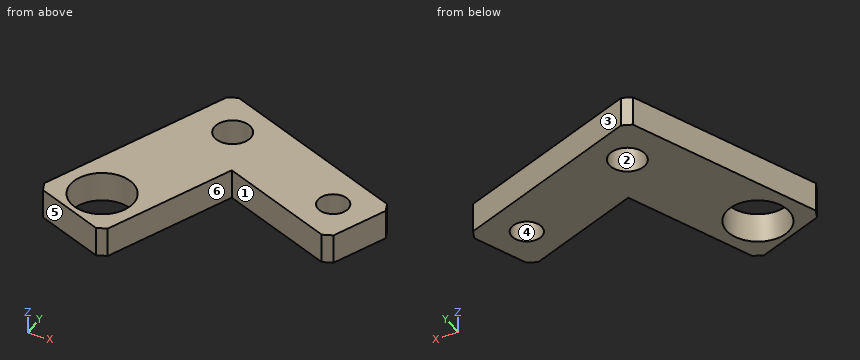
```python
from build123d import *

# Parameters (mm, degrees)
SKETCH_1_R      = 5.1
SKETCH_1_R_2    = 6.1
SKETCH_1_R_3    = 10.6
EXTRUDE_1_DEPTH = 10
CHAMFER_1_SIZE  = 2.5


with BuildPart() as part:
    # 草圖1 → 填料-伸長1 (new body)
    with BuildSketch(Plane.XY):
        Polygon((-42.684704159, 14.950876454), (26.753169389, -13.39311263), (17.305173028, -36.539070479), (-24.357551101, -19.532677029), (-43.253543823, -65.824592728), (-71.028693242, -54.486997094), align=None)
        with Locations((10.456192284, -20.242093374)):
            Circle(SKETCH_1_R, mode=Mode.SUBTRACT)
        with Locations((-33.52112763, -2.290900288)):
            Circle(SKETCH_1_R_2, mode=Mode.SUBTRACT)
        with Locations((-52.417120352, -48.582815986)):
            Circle(SKETCH_1_R_3, mode=Mode.SUBTRACT)
    extrude(amount=-EXTRUDE_1_DEPTH)

    # 導角1
    chamfer_1_edges = [part.edges().sort_by_distance(p)[0] for p in [
        (-42.684704159, 14.950876454, -5),
        (26.753169389, -13.39311263, -5),
        (17.305173028, -36.539070479, -5),
        (-43.253543823, -65.824592728, -5),
        (-71.028693242, -54.486997094, -5),
    ]]
    chamfer(chamfer_1_edges, length=CHAMFER_1_SIZE)


solid = part.part
```
Can you work these out from the model? Positions are in its coordinate system, mm. Face numbers are marked on the shaded views. A direction names the side the tool comes from. Give positions to 0.01 mm unless a question says otherwise; leave off trailing zeros. Loops run counter-clockwise (first coordinate to the right, second up) from the corner with the lowest first, then second, coordinate; pieces in that order, holes last. Notation, with made-up numbers: M 8.5,28 L 33.5,28 A34 cw 33.5,62 Z; hole C 70,-39.5 d3. An arc over 180 degrees is marked long. One line per item, written item: value.
(1) We'd pull the mould along Y, two halves only. Please class the marked faces 1, 2, 3 and 4: released by +Y, released by -Y, zero draft, split by the parting line, or undercut.
Returned:
face 1: released by -Y
face 2: undercut
face 3: released by +Y
face 4: undercut
(2) Suppose I cut it at A-A on y = -5.5. List the corners of the cut face in (x, z) for me, plus the area to 3 significant figures.
Returned:
outline: M -51.03,-10 L -38.71,-10 L -38.71,0 L -51.03,0 Z; M -28.33,-10 L 7.42,-10 L 7.42,0 L -28.33,0 Z
area: 481 mm^2
(3) Will these pins go through, and if not, where does the flat tip stop? pin 1 (4 mm diameter, centred on y = -32, z = -2, fed in from -X); pin 2 (4 mm diameter, centred on y = 3.5, z = -2.5, fed in from +X).
Returned:
pin 1: x = -62.67
pin 2: x = -9.73
(4) I need wall thicknesses on line 1 (X direction, y = -33.5, z = -1.5); line 2 (Y direction, x = 12, z = -4.25); line 3 (X direction, y = -30, z = -7.25). Which ranges of each line are inside material? Lowest first, please.
Returned:
line 1: -62.46 to -30.06, 9.86 to 18.55
line 2: -34.37 to -25.1, -15.38 to -7.37
line 3: -61.03 to -28.63, 1.29 to 19.97
(5) Suppose I cut it at B-B on x = 10.5. List the corners of the cut face in (y, z) for me, plus the area to 3 significant figures.
Returned:
outline: M -33.76,-10 L -25.34,-10 L -25.34,0 L -33.76,0 Z; M -15.14,-10 L -6.76,-10 L -6.76,0 L -15.14,0 Z
area: 168 mm^2
(6) Which directions (+Z, -Z, +X, -X, +Y, -Y) give clear straight access to the entire face, cutting with the end or side of a thin tool? Please do the marked faces 5 and 6.
Returned:
face 5: +Z, -Z, -X, -Y
face 6: +Z, -Z, -Y
(7) Suppose I cut it at D-D on x = -22.5. List the corners of the cut face in (y, z) for me, plus the area to 3 significant figures.
Returned:
outline: M -20.29,-10 L 6.71,-10 L 6.71,0 L -20.29,0 Z
area: 270 mm^2
(8) Suppose I cut it at C-C on z = -2. List the corners of the cut face in (x, y) for me.
Returned:
outline: M -70.08,-52.17 L -68.71,-55.43 L -45.57,-64.88 L -42.31,-63.51 L -24.36,-19.53 L 14.99,-35.59 L 18.25,-34.22 L 25.81,-15.71 L 24.44,-12.45 L -40.37,14.01 L -43.63,12.64 Z; hole C -52.42,-48.58 d21.2; hole C -33.52,-2.29 d12.2; hole C 10.46,-20.24 d10.2
